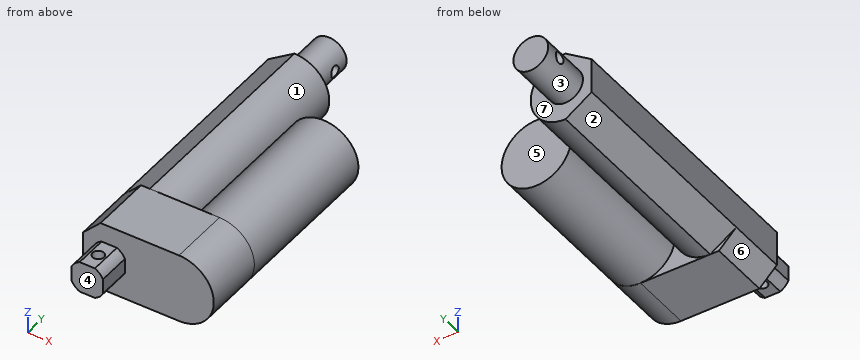
```python
from build123d import *

# Parameters (mm, degrees)
EXTRUDE_1_DEPTH     = 35
EXTRUDE_3_DEPTH     = 125
SKETCH_3_R          = 19.95
EXTRUDE_5_DEPTH     = 90
SKETCH_4_R          = 10
EXTRUDE_6_DEPTH     = 30
SKETCH_5_R          = 3.25
CUT_EXTRUDE_1_DEPTH = 30
EXTRUDE_START       = 19
EXTRUDE_7_DEPTH     = 19
CUT_EXTRUDE_2_REACH = 199.983
SKETCH_7_R          = 3.25


with BuildPart() as part:
    # Sketch 1 → Extrude 1 (new body)
    with BuildSketch(Plane(origin=(0, 0, 0), x_dir=(1, 0, 0), z_dir=(0, 1, 0))):
        with BuildLine():
            Line((-27.5, 10), (-17.5, 20))
            Line((-17.5, 20), (27.5, 20))
            ThreePointArc((27.5, 20), (47.5, 0), (27.5, -20))
            Line((27.5, -20), (-17.5, -20))
            Line((-17.5, -20), (-27.5, -10))
            Line((-27.5, -10), (-27.5, 10))
        make_face()
    extrude(amount=EXTRUDE_1_DEPTH)

    # Sketch 2 → Extrude 3 (add)
    with BuildSketch(Plane(origin=(0, 35, 0), x_dir=(1, 0, 0), z_dir=(0, 1, 0))):
        with BuildLine():
            Line((-12.5, 20), (-27.5, 10))
            Line((-27.5, 10), (-27.5, -10))
            Line((-27.5, -10), (-12.5, -20))
            ThreePointArc((-12.5, -20), (7.5, 0), (-12.5, 20))
        make_face()
    extrude(amount=EXTRUDE_3_DEPTH)

    # Sketch 3 → Extrude 5 (add)
    with BuildSketch(Plane(origin=(0, 35, 0), x_dir=(1, 0, 0), z_dir=(0, 1, 0))):
        with Locations(Location((27.5, 0, 0), (0, 0, 90))):
            Circle(SKETCH_3_R)
    extrude(amount=EXTRUDE_5_DEPTH)

    # Sketch 4 → Extrude 6 (add)
    with BuildSketch(Plane(origin=(0, 160, 0), x_dir=(1, 0, 0), z_dir=(0, 1, 0))):
        with Locations(Location((-12.5, 0, 0), (0, 0, 270))):
            Circle(SKETCH_4_R)
    extrude(amount=EXTRUDE_6_DEPTH)

    # Sketch 5 → Cut-Extrude 1 (cut)
    with BuildSketch(Plane(origin=(-27.5, 0, -27.5), x_dir=(0, 0, -1), z_dir=(1, 0, 0))):
        with Locations(Location((-27.5, 180, 0), (0, 0, 180))):
            Circle(SKETCH_5_R)
    extrude(amount=CUT_EXTRUDE_1_DEPTH, mode=Mode.SUBTRACT)

    # Sketch 6 → Extrude 7 (add)
    with BuildSketch(Plane.XZ.offset(EXTRUDE_START)):
        with BuildLine():
            Line((-16.858898944, -9), (-8.141101056, -9))
            ThreePointArc((-8.141101056, -9), (-5.428932188, -7.071067812), (-3.5, -4.358898944))
            Line((-3.5, -4.358898944), (-3.5, 4.358898944))
            ThreePointArc((-3.5, 4.358898944), (-5.428932188, 7.071067812), (-8.141101056, 9))
            Line((-8.141101056, 9), (-16.858898944, 9))
            ThreePointArc((-16.858898944, 9), (-19.571067812, 7.071067812), (-21.5, 4.358898944))
            Line((-21.5, 4.358898944), (-21.5, -4.358898944))
            ThreePointArc((-21.5, -4.358898944), (-19.571067812, -7.071067812), (-16.858898944, -9))
        make_face()
    extrude(amount=-EXTRUDE_7_DEPTH)

    # Sketch 7 → Cut-Extrude 2 (cut, up to next)
    with BuildSketch(Plane.XY.offset(9), mode=Mode.PRIVATE) as cut_extrude_2_sk1:
        with Locations((-12.5, -9.5)):
            Circle(SKETCH_7_R)
    cut_extrude_2_tool1 = extrude(cut_extrude_2_sk1.sketch, amount=-CUT_EXTRUDE_2_REACH, mode=Mode.PRIVATE) & part.part
    add(cut_extrude_2_tool1.solids().sort_by_distance((-12.5, -9.5, 9))[0], mode=Mode.SUBTRACT)


solid = part.part
```
Input: part model. Units: mm. Frame: model coordinates. Face numbers are marked on the shaded views. A direction names the side the tool comes from. Coordinates: 2 decimals unless noted, no trailing zeros. Write each loop counter-clockwise with the first axis right and the second up, starting at its lowest first coordinate (ties: lowest second). Pieces come first, ordered by that corner, then holes.
1) Section A-A on y = -9.5. Output: boundary loops of the cut face in (x, z), and give its area (3 significant figures).
2) Section D-D on y = 29. Output: boundary loops of the cut face in (x, z), and give its area (3 significant figures).
3) Set-up query: the marked faces 5, 6 and 7. Return all of +Z, -Z, +X, -X, +Y, -Y with unobstructed straight access to the full face (end or side cutting, diameter ignored); none if empty.
4) Section C-C on z = -15. Output: boundary loops of the cut face in (x, y), and give its area (3 significant figures).
5) Material intervals for line 1 along Y through (x, z) = (-12.5, -4.75); line 2 along Z through (x, y) = (-12, 180); line 3 along Y through (x, z) = (-12, -1), sorted ascending.
6) Pin query (flat end, axial travel): pin 1 Ø3 at (x, y) = (39, 6) entering from -Z; pin 2 Ø4 at (y, z) = (18.5, 6) entering from +X; pin 3 Ø6 at (y, z) = (125.5, 13.5) entering from -X. Return the tip coordinate at first contact, or that it passes through.
7) Section B-B on x = -6. Output: boundary loops of the cut face in (y, z), and give its area (3 significant figures).
8) Mould query, pull axis X, two halves, no side actions, for the marked faces 1, 2, 3 and 4. Classes: pulls with the +X half, pulls with the -X half, needs draft (parallel to the pull), parting line crosses it, or undercut.
Check result:
1. outline: (-21.5, -4.36) arc R10 ccw to (-16.86, -9) - (-15.75, -9) - (-15.75, 9) - (-16.86, 9) arc R10 ccw to (-21.5, 4.36) - close; (-9.25, -9) - (-8.14, -9) arc R10 ccw to (-3.5, -4.36) - (-3.5, 4.36) arc R10 ccw to (-8.14, 9) - (-9.25, 9) - close
1. area: 174 mm2
2. outline: (-27.5, -10) - (-17.5, -20) - (27.5, -20) arc R20 ccw to (27.5, 20) - (-17.5, 20) - (-27.5, 10) - close
2. area: 2,730 mm2
3. face 5: +Z, -Z, +X, +Y
3. face 6: -Z, -X, +Y, -Y
3. face 7: +Y
4. outline: (-22.5, 0) - (40.73, 0) - (40.73, 35) - (40.65, 35) - (40.65, 125) - (14.35, 125) - (14.35, 35) - (0.73, 35) - (0.73, 160) - (-20, 160) - (-20, 35) - (-22.5, 35) - close
4. area: 7,170 mm2
5. line 1: y = -19 to -12.75, -6.25 to 190
5. line 2: z = -9.99 to -3.25, 3.25 to 9.99
5. line 3: y = -19 to -12.71, -6.29 to 176.91, 183.09 to 190
6. pin 1: stops at z = -17.32
6. pin 2: stops at x = 47.1
6. pin 3: stops at x = -26.75
7. outline: (-19, -7.6) - (0, -7.6) - (0, -20) - (35, -20) - (35, -18.91) - (160, -18.91) - (160, -7.6) - (190, -7.6) - (190, 7.6) - (160, 7.6) - (160, 18.91) - (35, 18.91) - (35, 20) - (0, 20) - (0, 7.6) - (-19, 7.6) - close; hole circle Ø6.5 at (180, 0)
7. area: 6,840 mm2
8. face 1: undercut
8. face 2: pulls with the -X half
8. face 3: parting line crosses it
8. face 4: needs draft
